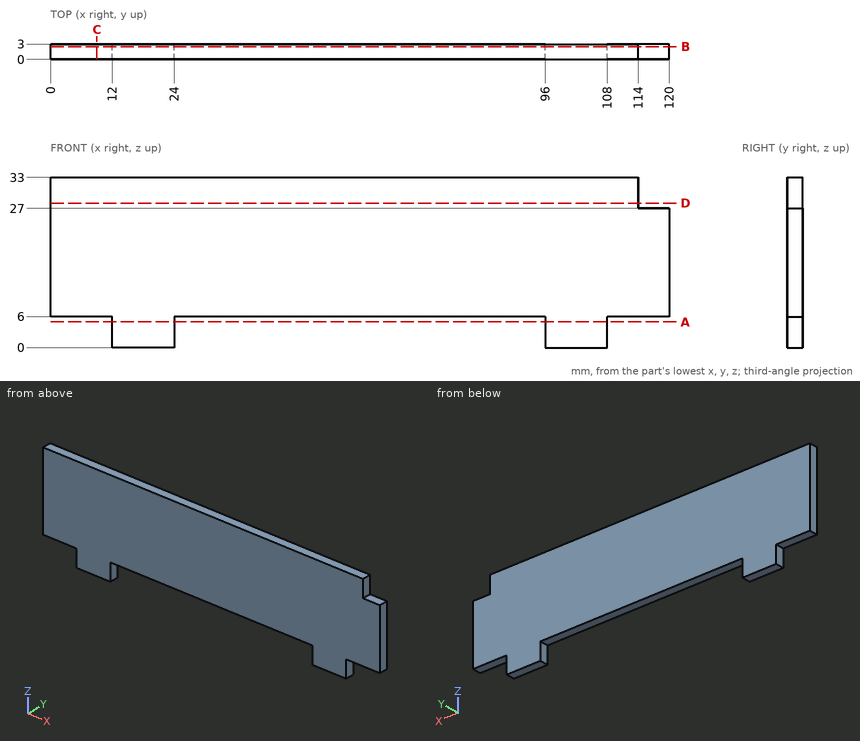
Can you work these out from the drawing? Everything is in mm from the part's minimum corner. Round coordinates to 2 decimals unless told otherwise and drop trailing zeros. Loops run counter-clockwise (first coordinate to the right, second up) from the corner with the lowest first, then second, coordinate; pieces in that order, holes last. Notation, with made-up numbers: M 32,17 L 39,17 A23 ccw 39,31 Z; hole C -18,44.25 d2. An arc over 180 degrees is marked long. Answer in a Markdown table with one row per item.
1. Please list where these lines run through material, in increasing order: line 1 (X direction, y = 0.45, z = 3.5); line 2 (Z direction, x = 61, y = 1.95). Write a range as from..to.
Established:
| item | result |
|---|---|
| line 1 | 12..24, 96..108 |
| line 2 | 6..33 |
2. I'm going to push flat-ended pins straight in: pin 1 Ø1.5 at (y, z) = (2, 29.5) entering from +X; pin 2 Ø0.9 at (y, z) = (1.5, 2.5) entering from -X; pin 3 Ø1.5 at (y, z) = (2, 2) entering from +X. Where does each tip first touch, or does it pass through?
Established:
| item | result |
|---|---|
| pin 1 | x = 114 |
| pin 2 | x = 12 |
| pin 3 | x = 108 |
3. If we section it at D-D, the plane z = 28: Please give me the cut outline in (x, y).
Established:
| item | result |
|---|---|
| outline | M 0,0 L 114,0 L 114,3 L 0,3 Z |
4. If we section it at A-A, the plane z = 5: Please give me the cut outline in (x, y).
Established:
| item | result |
|---|---|
| outline | M 12,0 L 24,0 L 24,3 L 12,3 Z; M 96,0 L 108,0 L 108,3 L 96,3 Z |
5. If we section it at B-B, the plane y = 2.5: Please give me the cut outline in (x, z), plus the area to 3 significant figures.
Established:
| item | result |
|---|---|
| outline | M 0,6 L 12,6 L 12,0 L 24,0 L 24,6 L 96,6 L 96,0 L 108,0 L 108,6 L 120,6 L 120,27 L 114,27 L 114,33 L 0,33 Z |
| area | 3,350 mm² |
6. If we section it at C-C, the plane x = 9: Please give me the cut outline in (y, z).
Established:
| item | result |
|---|---|
| outline | M 0,6 L 3,6 L 3,33 L 0,33 Z |
